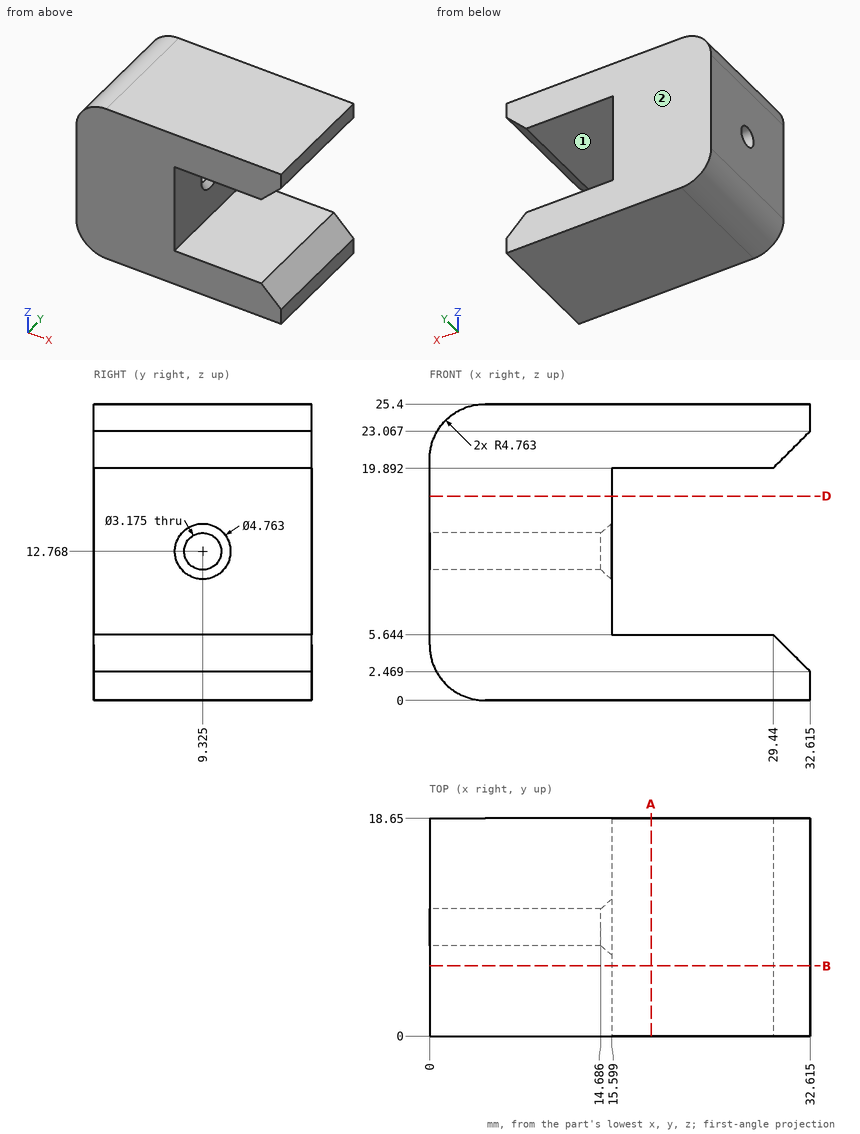
Design review of the part shown in the three views and the two pictorial views. Dimensions are in mm from the part's minimum x, y and z. A direction names the side the tool comes from. Round coordinates to 2 decimals unless told otherwise and drop trailing zeros. Loops run counter-clockwise (first coordinate to the right, second up) from the corner with the lowest first, then second, coordinate; pieces in that order, holes last. Notation, with made-up numbers: M 72,-27.75 L 126,-27.75 A23 cw 126,10.25 Z; hole C 29,-27 d8. An arc over 180 degrees is marked long. Put each result on its own line as item: value.
Q1. Machinability: for the marked faces 1 and 2, which of the approach directions +Z, -Z, +X, -X, +Y, -Y give a long, thin tool a straight path to every point of the face, cutting with its end or side? Answer none if there is none.
Result set:
face 1: +X, +Y, -Y
face 2: +Z, -Z, +X, -X, +Y
Q2. For pin 1 (4.5 mm diameter, centred on y = 6, z = 16.5, fed in from +X); pin 2 (8 mm diameter, centred on y = 9.5, z = 18.5, fed in from +X), all flat-tipped, find the tip position at first contact; note any pin that passes through.
Result set:
pin 1: stops at x = 15.6
pin 2: stops at x = 32.05
Q3. Consider section B-B, the plane y = 6. Give the boundary of the cut face in (x, z) (1 decimal).
Result set:
outline: M 0,4.8 A4.8 ccw 4.8,0 L 32.6,0 L 32.6,2.5 L 29.4,5.6 L 15.6,5.6 L 15.6,19.9 L 29.4,19.9 L 32.6,23.1 L 32.6,25.4 L 4.8,25.4 A4.8 ccw 0,20.6 Z
Q4. Consider section D-D, the plane z = 17.5. Give the boundary of the cut face in (x, y), then the cut area to 3 significant figures.
Result set:
outline: M 0,0 L 15.6,0 L 15.6,18.65 L 0,18.65 Z
area: 291 mm²
Q5. To check wall thickness, follow L1, parallel to Z at x = 19, y = 6; L2, parallel to Y at x = 1.5, z = 12.75; L3, parallel to X at y = 15, z = 19.25. State the ranges of each line that lie inside material, in increasing order.
Result set:
L1: z = 0 to 5.64, 19.89 to 25.4
L2: y = 0 to 7.74, 10.91 to 18.65
L3: x = 0 to 15.6
Q6. Consider section A-A, the plane x = 19. Give the boundary of the cut face in (y, z).
Result set:
outline: M 0,0 L 18.65,0 L 18.65,5.64 L 0,5.64 Z; M 0,19.89 L 18.65,19.89 L 18.65,25.4 L 0,25.4 Z
